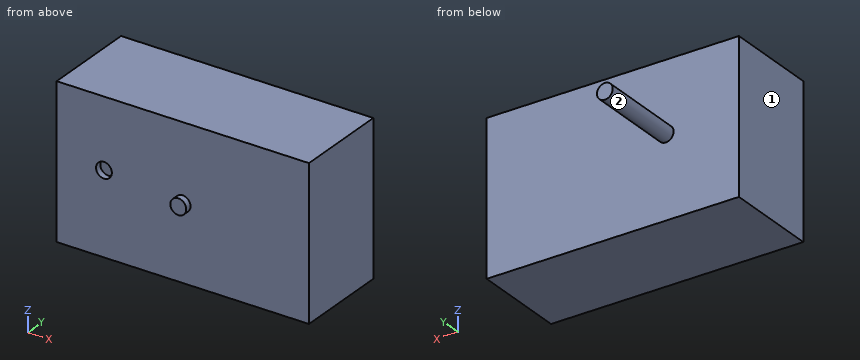
from build123d import *

# Parameters (mm, degrees)
SKETCH1_W                 = 101.6
SKETCH1_H                 = 60.96
SKETCH1_R                 = 3.175
BOSS_EXTRUDE1_DEPTH       = 2.54
SKETCH2_R                 = 3.197303881
CUT_EXTRUDE1_DEPTH        = 2.54
BOSS_EXTRUDE2_DEPTH       = 30.48
BOSS_EXTRUDE2_DEPTH_BACK  = 5.08
SKETCH3_R                 = 3.197303881
SKETCH6_W                 = 2.54
SKETCH6_H                 = 60.96
BOSS_EXTRUDE10_DEPTH      = 33.02
SKETCH7_W                 = 96.52
SKETCH7_H                 = 2.54
BOSS_EXTRUDE11_DEPTH      = 33.02
SKETCH9_W                 = 101.6
SKETCH9_H                 = 60.96
BOSS_EXTRUDE12_DEPTH      = 2.54
BOSS_EXTRUDE13_DEPTH      = 36.068
BOSS_EXTRUDE13_DEPTH_BACK = 12.7
SKETCH10_R                = 3.175


with BuildPart() as part:
    # Sketch1 → Boss-Extrude1 (new body)
    with BuildSketch(Plane(origin=(0, 0, 0), x_dir=(1, 0, 0), z_dir=(0, 1, 0))):
        Rectangle(SKETCH1_W, SKETCH1_H)
        with Locations(Location((-31.75, -2.54, 0), (0, 0, 270))):
            Circle(SKETCH1_R, mode=Mode.SUBTRACT)
    extrude(amount=BOSS_EXTRUDE1_DEPTH)

    # Sketch2 → Cut-Extrude1 (cut)
    with BuildSketch(Plane(origin=(0, 2.54, 0), x_dir=(1, 0, 0), z_dir=(0, 1, 0))):
        with Locations(Location((-0.087463015, 0.456757565, 0), (0, 0, 270))):
            Circle(SKETCH2_R)
    extrude(amount=-CUT_EXTRUDE1_DEPTH, mode=Mode.SUBTRACT)

    # Sketch3 → Boss-Extrude2 (add, two sides: drawn at the far end of the back side and taken through both)
    with BuildSketch(Plane(origin=(0, 2.54, 0), x_dir=(1, 0, 0), z_dir=(0, 1, 0)).offset(-BOSS_EXTRUDE2_DEPTH_BACK)):
        with Locations(Location((-0.087463015, 0.456757565, 0), (0, 0, 270))):
            Circle(SKETCH3_R)
    extrude(amount=BOSS_EXTRUDE2_DEPTH + BOSS_EXTRUDE2_DEPTH_BACK)

    # Sketch6 → Boss-Extrude10 (add)
    with BuildSketch(Plane(origin=(0, 2.54, 0), x_dir=(1, 0, 0), z_dir=(0, 1, 0))):
        with Locations((-49.53, 0)):
            Rectangle(SKETCH6_W, SKETCH6_H)
        with Locations((49.53, 0)):
            Rectangle(SKETCH6_W, SKETCH6_H)
    extrude(amount=BOSS_EXTRUDE10_DEPTH)

    # Sketch7 → Boss-Extrude11 (add)
    with BuildSketch(Plane(origin=(0, 2.54, 0), x_dir=(1, 0, 0), z_dir=(0, 1, 0))):
        with Locations((0, 29.21)):
            Rectangle(SKETCH7_W, SKETCH7_H)
        with Locations((0, -29.21)):
            Rectangle(SKETCH7_W, SKETCH7_H)
    extrude(amount=BOSS_EXTRUDE11_DEPTH)

    # Sketch9 → Boss-Extrude12 (add)
    with BuildSketch(Plane(origin=(0, 35.56, 0), x_dir=(1, 0, 0), z_dir=(0, 1, 0))):
        Rectangle(SKETCH9_W, SKETCH9_H)
    extrude(amount=BOSS_EXTRUDE12_DEPTH)

    # Sketch10 → Boss-Extrude13 (add, two sides: drawn at the far end of the back side and taken through both)
    with BuildSketch(Plane(origin=(0, 38.1, 0), x_dir=(1, 0, 0), z_dir=(0, 1, 0)).offset(-BOSS_EXTRUDE13_DEPTH_BACK)):
        with Locations(Location((-21.325114791, -2.320034183, 0), (0, 0, 270))):
            Circle(SKETCH10_R)
    extrude(amount=BOSS_EXTRUDE13_DEPTH + BOSS_EXTRUDE13_DEPTH_BACK)


solid = part.part
Design review of the part built by this model. Coordinates are the model's own, in mm. Face numbers are marked on the shaded views. A direction names the side the tool comes from. Round coordinates to 2 decimals unless told otherwise and drop trailing zeros. Loops run counter-clockwise (first coordinate to the right, second up) from the corner with the lowest first, then second, coordinate; pieces in that order, holes last. Notation, with made-up numbers: (15, 79.5) -> (44, 79.5) arc R15 cw to (44, 93.5) -> close; hole circle Ø6 at (7.5, 1.5). An arc over 180 degrees is marked (long way). Use one line per item in the form item = value. Start each with the question number.
Q1. We need section A-A on y = 19.5. Give the boundary of the cut face in (x, z).
Q2. We need section C-C on z = -8. Give the boundary of the cut face in (x, y).
Q3. We need section B-B on y = 30.5. Give the boundary of the cut face in (x, z) (3 decimals).
Q4. Wall thickness on line 1 along X through (y, z) = (1.4, 2.54) (3 decimals); line 2 along Z through (x, y) = (19, 24.5); line 3 along X through (y, z) = (14, 26.5): over which ranges is each line inside the solid? List them lowest first. Write a range as [from, to].
Q5. Machinability: for the marked faces 1 and 2, which of the approach directions +Z, -Z, +X, -X, +Y, -Y give a long, thin tool a straight path to every point of the face, cutting with its end or side? Answer none if there is none.
Q6. We need section D-D on x = 13.5. Give the boundary of the cut face in (y, z), then the cut area to 3 significant figures.
Q7. For pin 1 Ø10 at (x, z) = (-36, 6) entering from -Y; pin 2 Ø8 at (x, z) = (36, -9) entering from +Y; pin 3 Ø10 at (y, z) = (46, -10) entering from -X, all flat-tipped, find the tip position at first contact; note any pin that passes through.
Calculated:
q1.outline = (-50.8, -30.48) -> (50.8, -30.48) -> (50.8, 30.48) -> (-50.8, 30.48) -> close; circle Ø6.39 at (-0.09, -0.46); hole (-48.26, -27.94) -> (48.26, -27.94) -> (48.26, 27.94) -> (-48.26, 27.94) -> close
q2.outline = (-50.8, 0) -> (50.8, 0) -> (50.8, 38.1) -> (-50.8, 38.1) -> close; hole (-48.26, 2.54) -> (48.26, 2.54) -> (48.26, 35.56) -> (-48.26, 35.56) -> close
q3.outline = (-50.8, -30.48) -> (50.8, -30.48) -> (50.8, 30.48) -> (-50.8, 30.48) -> close; circle Ø6.35 at (-21.325, 2.32); circle Ø6.395 at (-0.087, -0.457); hole (-48.26, -27.94) -> (48.26, -27.94) -> (48.26, 27.94) -> (-48.26, 27.94) -> close
q4.line_1 = [-50.8, -34.925], [-28.575, 50.8]
q4.line_2 = [-30.48, -27.94], [27.94, 30.48]
q4.line_3 = [-50.8, -48.26], [48.26, 50.8]
q5.face_1 = +Z, -Z, -X, +Y, -Y
q5.face_2 = +Y
q6.outline = (0, -30.48) -> (38.1, -30.48) -> (38.1, 30.48) -> (0, 30.48) -> close; hole (2.54, -27.94) -> (35.56, -27.94) -> (35.56, 27.94) -> (2.54, 27.94) -> close
q6.area = 477 mm²
q7.pin_1 = 0
q7.pin_2 = 38.1
q7.pin_3 = through
